Design review of the part shown in the three views and the two pictorial views. Dimensions are in mm from the part's minimum x, y and z. A direction names the side the tool comes from. Round coordinates to 2 decimals unless told otherwise and drop trailing zeros. Write each loop counter-clockwise with the first axis right and the second up, starting at its lowest first coordinate (ties: lowest second). Pieces come first, ordered by that corner, then holes. Notation, with made-up numbers: (41, -22.5) -> (83, -22.5) arc R9 ccw to (83, -17.5) -> close; hole circle Ø3 at (-37, -15). An arc over 180 degrees is marked (long way). Answer as a JSON object with one key per item and string values. Group by question number.
1) Insertion check: pin 1 Ø2 at (x, z) = (6.82, 6.82) entering from +Y; pin 2 Ø8 at (x, y) = (12.5, 5.5) entering from -Z (1 decimal); pin 3 Ø3 at (x, z) = (27.68, 6.82) entering from +Y (3 decimals); pin 4 Ø3 at (x, z) = (27.68, 27.68) entering from -Y (3 decimals). Each pin has a flat end and moves straight along its axis. Give the tip position at first contact, or say it passes through.
2) We need section A-A, the plane x = 17.25. Write out the cut boundary in (y, z) (3 decimals), then the cut area to 3 significant figures.
3) We need section B-B, the plane z = 17.25. Write out the cut boundary in (x, y) (3 decimals), then the cut area to 3 significant figures.
4) To check wall thickness, follow probe 1 along X at (y, z) = (26.5, 17.25); probe 2 along Y at (x, z) = (31.5, 11.5) (3 decimals); probe 3 along Z at (x, y) = (17.5, 23.25) (1 decimal). State the ranges of each line that lie inside material, in increasing order. Write a range as [from, to].
5) We need section D-D, the plane y = 25. Count the separate pieces of the cut face and the enclosed holes in it.
6) Machinability: for the marked faces 3 and 4, which of the approach directions +Z, -Z, +X, -X, +Y, -Y give a long, thin tool a straight path to every point of the face, cutting with its end or side? Answer none if there is none.
7) We need section C-C, the plane x = 3. Write out the cut boundary in (y, z) (1 decimal).
8) Mouldability with a two-part tool opening along X and no side actions: class the marked faces 1 and 2 as pulls with the +X half, pulls with the -X half, needs draft (parallel to the pull), parting line crosses it, or undercut.
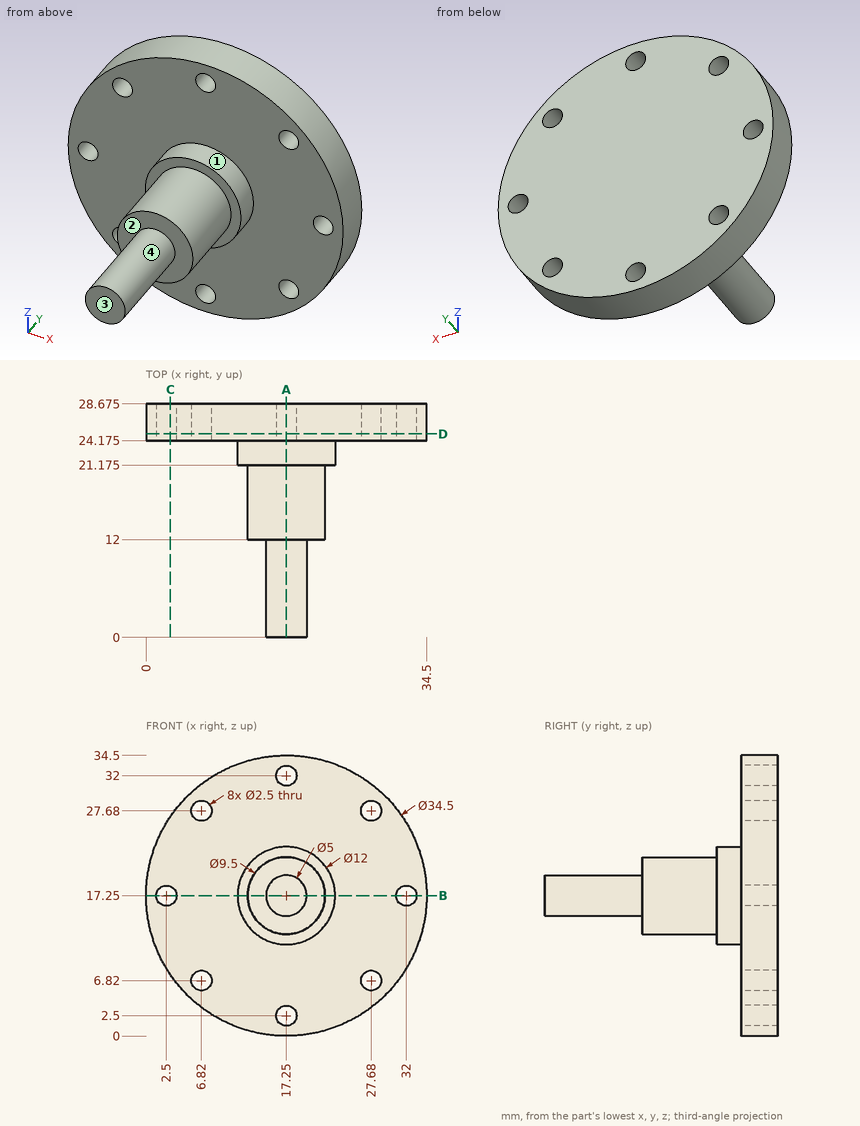
Here are the results:
{
 "1": {"pin 1": "passes through", "pin 2": "stops at z = 14.9", "pin 3": "stops at y = 28.675", "pin 4": "stops at y = 24.175"},
 "2": {"outline": "(0, 14.75) -> (12, 14.75) -> (12, 12.5) -> (21.175, 12.5) -> (21.175, 11.25) -> (24.175, 11.25) -> (24.175, 3.75) -> (28.675, 3.75) -> (28.675, 30.75) -> (24.175, 30.75) -> (24.175, 23.25) -> (21.175, 23.25) -> (21.175, 22) -> (12, 22) -> (12, 19.75) -> (0, 19.75) -> close; (24.175, 0) -> (28.675, 0) -> (28.675, 1.25) -> (24.175, 1.25) -> close; (24.175, 33.25) -> (28.675, 33.25) -> (28.675, 34.5) -> (24.175, 34.5) -> close", "area": "316 mm^2"},
 "3": {"outline": "(0, 24.175) -> (1.25, 24.175) -> (1.25, 28.675) -> (0, 28.675) -> close; (3.75, 24.175) -> (11.25, 24.175) -> (11.25, 21.175) -> (12.5, 21.175) -> (12.5, 12) -> (14.75, 12) -> (14.75, 0) -> (19.75, 0) -> (19.75, 12) -> (22, 12) -> (22, 21.175) -> (23.25, 21.175) -> (23.25, 24.175) -> (30.75, 24.175) -> (30.75, 28.675) -> (3.75, 28.675) -> close; (33.25, 24.175) -> (34.5, 24.175) -> (34.5, 28.675) -> (33.25, 28.675) -> close", "area": "316 mm^2"},
 "4": {"probe 1": "x = [0, 1.25], [3.75, 30.75], [33.25, 34.5]", "probe 2": "y = [24.175, 28.675]", "probe 3": "z = [11.3, 23.2]"},
 "5": {"separate pieces": "1", "enclosed holes": "8"},
 "6": {"face 3": "+Z, -Z, +X, -X, -Y", "face 4": "-Y"},
 "7": {"outline": "(24.2, 7.5) -> (28.7, 7.5) -> (28.7, 16.1) -> (24.2, 16.1) -> close; (24.2, 18.4) -> (28.7, 18.4) -> (28.7, 27) -> (24.2, 27) -> close"},
 "8": {"face 1": "parting line crosses it", "face 2": "needs draft"}
}
